Could you check a few things on this model? Use its own coordinates, in mm. A direction names the side the tool comes from. Round coordinates to 2 decimals unless told otherwise and drop trailing zeros. Order: outer loops, then holes, each group sorted by start corner. A loop starts at its lowest first (then second) coordinate and runs counter-clockwise, first axis right, second up.
```python
from build123d import *

# Parameters (mm, degrees)
SKETCH_1_R      = 1.25
EXTRUDE_1_DEPTH = 3


with BuildPart() as part:
    # 草图1 → 凸台-拉伸1 (new body)
    with BuildSketch(Plane.XY):
        with BuildLine():
            ThreePointArc((3.5, 7), (0, 3.5), (-3.5, 7))
            Line((-3.5, 7), (-3.5, 16.63580476))
            ThreePointArc((-3.5, 16.63580476), (-12.02081528, 12.02081528), (-16.63580476, 3.5))
            Line((-16.63580476, 3.5), (-7, 3.5))
            ThreePointArc((-7, 3.5), (-4.525126266, 2.474873734), (-3.5, 0))
            ThreePointArc((-3.5, 0), (-4.525126266, -2.474873734), (-7, -3.5))
            Line((-7, -3.5), (-16.63580476, -3.5))
            ThreePointArc((-16.63580476, -3.5), (-12.02081528, -12.02081528), (-3.5, -16.63580476))
            Line((-3.5, -16.63580476), (-3.5, -7))
            ThreePointArc((-3.5, -7), (0, -3.5), (3.5, -7))
            Line((3.5, -7), (3.5, -16.63580476))
            ThreePointArc((3.5, -16.63580476), (12.02081528, -12.02081528), (16.63580476, -3.5))
            Line((16.63580476, -3.5), (7, -3.5))
            ThreePointArc((7, -3.5), (3.5, 0), (7, 3.5))
            Line((7, 3.5), (16.63580476, 3.5))
            ThreePointArc((16.63580476, 3.5), (12.02081528, 12.02081528), (3.5, 16.63580476))
            Line((3.5, 16.63580476), (3.5, 7))
        make_face()
        Circle(SKETCH_1_R, mode=Mode.SUBTRACT)
    extrude(amount=EXTRUDE_1_DEPTH)


solid = part.part
```
Q1. Imagine slicing it at A-A, the plane x = -8. Please give me the cut outline in (y, z).
Q2. We'd pull the mould along Y, two halves only. Please class faces 1 (the flat face through (-3.5, 12, 1)), 2 (the cylindrical face through (12.12, 11.92, 1.48)), 3 (the flat face through (-12, 3.5, 1)): released by +Y, released by -Y, zero draft, split by the parting line, or undercut.
Q3. For P1, Ø1.5, axis at x = -10.5, z = 2.5, coming from the +Y side; P2, Ø8, axis at x = 11.5, y = -2, coming from the +Z side; P3, Ø1.5, axis at x = -13.5, z = 1, coming from the +Y side; P4, Ø0.9, axis at y = -9.5, z = 2, coming from the -X side, each with a flat end and sliding along its axis, tell me the tip position at first contact or that it passes through.
Q4. Imagine slicing it at D-D, the plane y = -3. Please give me the cut outline in (x, z), then the cut area to 3 significant figures.
Q5. I need wall thicknesses on L1, parallel to Y at x = 0, z = 2.05; L2, parallel to Y at x = 12, z = 1.8; L3, parallel to X at y = -8.5, z = 2.75. Which ranges of each line are inside material? Lowest first, please.
Q6. Imagine slicing it at B-B, the plane y = 15. Please give me the cut outline in (x, z).
Q7. For faces 4 (the flat face through (-12, -3.5, 1)), 5 (the flat face through (3, 0, 0)), 6 (the flat face through (12, -3.5, 1)), 7 (the flat face through (3.5, 12, 1)), 8 (the flat face through (3.5, -12, 1)), which set-ups out of +Z, -Z, +X, -X, +Y, -Y let a thin tool reach every point of the face, with its end or its side?
Q8. Imagine slicing it at C-C, the plane z = 1.75. Please give me the cut outline in (x, y).
Filled in:
1. outline: (-15, 0) - (-3.5, 0) - (-3.5, 3) - (-15, 3) - close; (3.5, 0) - (15, 0) - (15, 3) - (3.5, 3) - close
2. face 1: zero draft
2. face 2: released by +Y
2. face 3: undercut
3. P1: stops at y = 13.93
3. P2: stops at z = 3
3. P3: stops at y = 11.24
3. P4: stops at x = -14.39
4. outline: (-5.2, 0) - (5.2, 0) - (5.2, 3) - (-5.2, 3) - close
4. area: 31.2 mm2
5. L1: y = -3.5 to -1.25, 1.25 to 3.5
5. L2: y = -12.04 to -3.5, 3.5 to 12.04
5. L3: x = -14.72 to -3.5, 3.5 to 14.72
6. outline: (-8, 0) - (-3.5, 0) - (-3.5, 3) - (-8, 3) - close; (3.5, 0) - (8, 0) - (8, 3) - (3.5, 3) - close
7. face 4: +Z, -Z, -X
7. face 5: -Z, +X, -X, +Y, -Y
7. face 6: +Z, -Z, +X
7. face 7: +Z, -Z, +Y
7. face 8: +Z, -Z, -Y
8. outline: (-16.64, -3.5) arc R17 ccw to (-3.5, -16.64) - (-3.5, -7) arc R3.5 cw to (3.5, -7) - (3.5, -16.64) arc R17 ccw to (16.64, -3.5) - (7, -3.5) arc R3.5 cw to (7, 3.5) - (16.64, 3.5) arc R17 ccw to (3.5, 16.64) - (3.5, 7) arc R3.5 cw to (-3.5, 7) - (-3.5, 16.64) arc R17 ccw to (-16.64, 3.5) - (-7, 3.5) arc R3.5 cw to (-7, -3.5) - close; hole circle Ø2.5 at (0, 0)
